Geometry: final body of the model. Coordinates: model frame, mm. Face numbers are marked on the shaded views. A direction names the side the tool comes from. Round coordinates to 2 decimals unless told otherwise and drop trailing zeros. Loops run counter-clockwise (first coordinate to the right, second up) from the corner with the lowest first, then second, coordinate; pieces in that order, holes last. Notation, with made-up numbers: (73, 56.25) -> (83, 56.25) arc R22 cw to (83, 81.25) -> close; hole circle Ø8 at (61.5, 57.25). An arc over 180 degrees is marked (long way). Answer in a Markdown table with one row per item.
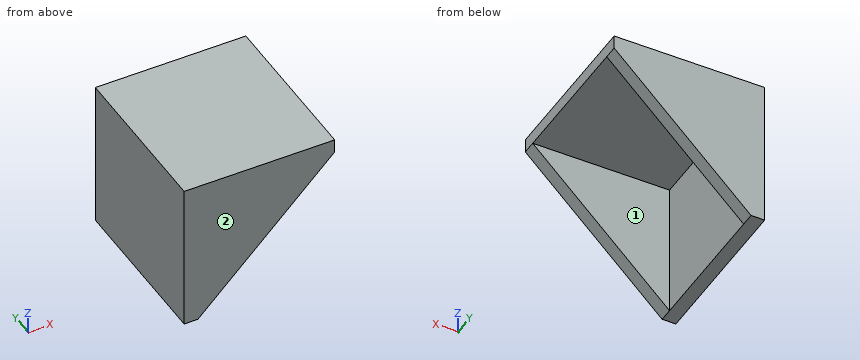
```python
from build123d import *

# Parameters (mm, degrees)
F2_W     = 5
F2_H     = 50
F2_W_2   = 50
F3_DEPTH = 5
F4_DEPTH = 50
F6_DEPTH = 60.001


with BuildPart() as f3:
    # F2 (on Top) → F3 (new body)
    with BuildSketch(Plane.XY):
        Polygon((-30, 25), (-25, 25), (25, 25), (25, 30), (-30, 30), align=None)
        with Locations((-27.5, 0)):
            Rectangle(F2_W, F2_H)
        Rectangle(F2_W_2, F2_H)
        Polygon((25, -25), (-25, -25), (-30, -25), (-30, -30), (25, -30), align=None)
    extrude(amount=F3_DEPTH)

    # F2 (on Top) → F4 (join)
    with BuildSketch(Plane.XY):
        Polygon((25, -25), (-25, -25), (-30, -25), (-30, -30), (25, -30), align=None)
        Polygon((-30, 25), (-25, 25), (25, 25), (25, 30), (-30, 30), align=None)
        with Locations((-27.5, 0)):
            Rectangle(F2_W, F2_H)
    extrude(amount=-F4_DEPTH)

    # F5 (on face) → F6 (cut, through all)
    with BuildSketch(Plane(origin=(0, 30, 0), x_dir=(-1, 0, 0), z_dir=(0, 1, 0))):
        Polygon((25, -50), (-25, 0), (-25, -50), align=None)
    extrude(amount=-F6_DEPTH, mode=Mode.SUBTRACT)


solid = f3.part
```
Item 1: Cut plane B-B (x = -15). Output: boundary loops of the cut face in (y, z).
Answer:
| item | result |
|---|---|
| outline | (-30, -40) -> (-25, -40) -> (-25, 0) -> (25, 0) -> (25, -40) -> (30, -40) -> (30, 5) -> (-30, 5) -> close |
Item 2: Cut plane A-A (z = -1). Output: boundary loops of the cut face in (x, y).
Answer:
| item | result |
|---|---|
| outline | (-30, -30) -> (24, -30) -> (24, -25) -> (-25, -25) -> (-25, 25) -> (24, 25) -> (24, 30) -> (-30, 30) -> close |
Item 3: Reachability of the marked faces 1 and 2 from +Z, -Z, +X, -X, +Y, -Y: full face, straight path, thin tool, end or side. Return the list, or none.
Answer:
| item | result |
|---|---|
| face 1 | -Z, +X |
| face 2 | +Z, -Z, +X, -X, -Y |
Item 4: Cut plane C-C (y = -18). Output: boundary loops of the cut face in (x, z), then the cut area to 3 significant figures.
Answer:
| item | result |
|---|---|
| outline | (-30, -50) -> (-25, -50) -> (-25, 0) -> (25, 0) -> (25, 5) -> (-30, 5) -> close |
| area | 525 mm² |
Item 5: Line query: probe 1 along Y at (x, z) = (-16.5, -11.5); probe 2 along Z at (x, y) = (-24, -20); probe 3 along X at (y, z) = (-18.5, -43). Output: solid intervals per line, ascending. Write a range as [from, to].
Answer:
| item | result |
|---|---|
| probe 1 | y = [-30, -25], [25, 30] |
| probe 2 | z = [0, 5] |
| probe 3 | x = [-30, -25] |
Item 6: Pin query (flat end, axial travel): pin 1 Ø2 at (x, y) = (-2.5, -10.5) entering from -Z; pin 2 Ø15 at (y, z) = (10, -21.5) entering from +X; pin 3 Ø5 at (x, z) = (-8.5, -35.5) entering from +Y. Return the tip coordinate at first contact, or that it passes through.
Answer:
| item | result |
|---|---|
| pin 1 | stops at z = 0 |
| pin 2 | stops at x = -25 |
| pin 3 | stops at y = 30 |
